from build123d import *

# Parameters (mm, degrees)
F1_DEPTH = 8
F2_W     = 118.303065
F2_H     = 130
F3_DEPTH = 2.5
F4_R     = 2.5
F5_DEPTH = 5


with BuildPart() as f1:
    # F0 (on Top) → F1 (new body)
    with BuildSketch(Plane.XY):
        with BuildLine():
            Line((-73, 0), (0, 0))
            Line((0, 0), (73, 0))
            ThreePointArc((73, 0), (74.414214, 0.585786), (75, 2))
            Line((75, 2), (75, 7.775523))
            ThreePointArc((75, 7.775523), (73.927452, 10.50133), (71.284988, 11.765358))
            Line((71.284988, 11.765358), (60.101284, 12.564194))
            ThreePointArc((60.101284, 12.564194), (55.064204, 13.247802), (50.154497, 14.564715))
            Line((50.154497, 14.564715), (16.502155, 25.927844))
            ThreePointArc((16.502155, 25.927844), (13.721064, 27.682003), (12.047716, 30.512454))
            ThreePointArc((12.047716, 30.512454), (11.731046, 31.611641), (11.450465, 32.720588))
            ThreePointArc((11.450465, 32.720588), (9.052802, 46.392588), (8.25, 60.25))
            Line((8.25, 60.25), (8.25, 92.25))
            ThreePointArc((8.25, 92.25), (9.052802, 106.107412), (11.450465, 119.779412))
            ThreePointArc((11.450465, 119.779412), (11.814902, 121.192928), (12.237963, 122.590018))
            ThreePointArc((12.237963, 122.590018), (13.860893, 125.287212), (16.501569, 127.000568))
            Line((16.501569, 127.000568), (35.134496, 133.776176))
            ThreePointArc((35.134496, 133.776176), (36.60869, 134.936374), (37.105525, 136.745369))
            Line((37.105525, 136.745369), (36.057795, 157.7))
            ThreePointArc((36.057795, 157.7), (35.86861, 159.074474), (35.444795, 160.395592))
            ThreePointArc((35.444795, 160.395592), (31.086723, 166.367805), (24.508944, 169.743151))
            ThreePointArc((24.508944, 169.743151), (18.300743, 170.974097), (12.006736, 171.63927))
            ThreePointArc((12.006736, 171.63927), (6.006077, 171.909797), (0, 172))
            ThreePointArc((0, 172), (-6.006077, 171.909797), (-12.006736, 171.63927))
            ThreePointArc((-12.006736, 171.63927), (-18.300743, 170.974097), (-24.508944, 169.743151))
            ThreePointArc((-24.508944, 169.743151), (-31.086723, 166.367805), (-35.444795, 160.395592))
            ThreePointArc((-35.444795, 160.395592), (-35.86861, 159.074474), (-36.057795, 157.7))
            Line((-36.057795, 157.7), (-37.105525, 136.745369))
            ThreePointArc((-37.105525, 136.745369), (-36.60869, 134.936374), (-35.134496, 133.776176))
            Line((-35.134496, 133.776176), (-16.501569, 127.000568))
            ThreePointArc((-16.501569, 127.000568), (-13.860893, 125.287212), (-12.237963, 122.590018))
            ThreePointArc((-12.237963, 122.590018), (-11.814902, 121.192928), (-11.450465, 119.779412))
            ThreePointArc((-11.450465, 119.779412), (-9.052802, 106.107412), (-8.25, 92.25))
            Line((-8.25, 92.25), (-8.25, 60.25))
            ThreePointArc((-8.25, 60.25), (-9.052802, 46.392588), (-11.450465, 32.720588))
            ThreePointArc((-11.450465, 32.720588), (-11.731046, 31.611641), (-12.047716, 30.512454))
            ThreePointArc((-12.047716, 30.512454), (-13.721064, 27.682003), (-16.502155, 25.927844))
            Line((-16.502155, 25.927844), (-50.154497, 14.564715))
            ThreePointArc((-50.154497, 14.564715), (-55.064204, 13.247802), (-60.101284, 12.564194))
            Line((-60.101284, 12.564194), (-71.284988, 11.765358))
            ThreePointArc((-71.284988, 11.765358), (-73.927452, 10.50133), (-75, 7.775523))
            Line((-75, 7.775523), (-75, 2))
            ThreePointArc((-75, 2), (-74.414214, 0.585786), (-73, 0))
        make_face()
    extrude(amount=F1_DEPTH)

    # F2 (on face) → F3 (cut)
    with BuildSketch(Plane.XY.offset(8)):
        with Locations((59.151532, 83)):
            Rectangle(F2_W, F2_H)
    extrude(amount=-F3_DEPTH, mode=Mode.SUBTRACT)

    # F4 (on face) → F5 (join)
    with BuildSketch(Plane.XY.offset(8)):
        with Locations((0, 10)):
            Circle(F4_R)
        with Locations((-13, 148)):
            Circle(F4_R)
    extrude(amount=F5_DEPTH)


solid = f1.part
CAD build for the part. Positions are in the model's coordinates, mm. A direction names the side the tool comes from. Give positions to 0.01 mm unless a question says otherwise; leave off trailing zeros. Write each loop counter-clockwise with the first axis right and the second up, starting at its lowest first coordinate (ties: lowest second). Pieces come first, ordered by that corner, then holes. Notation, with made-up numbers: (57, 66.5) - (105, 66.5) arc R6 cw to (105, 75.5) - close; hole circle Ø3 at (81, -35.5). An arc over 180 degrees is marked (long way). Put each result on its own line as item: value.
(1) Saw through at D-D (y = 22.5). List the corners of the cut face in (x, z).
Working result:
outline: (-26.65, 0) - (26.65, 0) - (26.65, 5.5) - (0, 5.5) - (0, 8) - (-26.65, 8) - close
(2) Saw through at C-C (y = 141.5). List the corners of the cut face in (x, z).
Working result:
outline: (-36.87, 0) - (36.87, 0) - (36.87, 5.5) - (0, 5.5) - (0, 8) - (-36.87, 8) - close
(3) Saw through at A-A (z = 10.75). List the corners of the cut face in (x, y).
Working result:
outline: circle Ø5 at (-13, 148); circle Ø5 at (0, 10)
(4) Pull direction Y, two halves, no side cores. Call faces 4 (the cylindrical face through (-0.54, 7.56, 10.46)), 5 (the flat face through (-65.61, 12.17, 3.94)), 6 (the flat face through (33.56, 20.17, 3.06)): released by +Y, released by -Y, zero draft, split by the parting line, or undercut.
Working result:
face 4: split by the parting line
face 5: released by +Y
face 6: undercut
(5) Saw through at B-B (x = -28). List the corners of the cut face in (y, z).
Working result:
outline: (0, 0) - (22.05, 0) - (22.05, 8) - (0, 8) - close; (131.18, 0) - (168.44, 0) - (168.44, 8) - (131.18, 8) - close
(6) Wall check: L1, parallel to Y at x = 12, z = 6.5; L2, parallel to Z at x = 6, y = 149; L3, parallel to Y at x = 16, z = 5. Give the ranges that are in metal, low to high.
Working result:
L1: 0 to 18, 148 to 171.64
L2: 0 to 8
L3: 0 to 26.12, 126.8 to 171.28
(7) Drop flat-ended pins along their axis: pin 1 Ø1.6 at (y, z) = (83.5, 3.5) entering from +X; pin 2 Ø2 at (x, z) = (12, 7) entering from +Y; pin 3 Ø1 at (y, z) = (91, 9) entering from +X; pin 4 Ø4 at (y, z) = (117.5, 4.5) entering from -X. Give the stop position or say it passes through.
Working result:
pin 1: x = 8.25
pin 2: y = 171.7
pin 3: through
pin 4: x = -11.38
(8) Tool access for faces 1 (the cylindrical face through (55.134, 13.234, 3.944)), 2 (the flat face through (8.25, 76, 3)), 3 (the flat face through (-33.093, 20.326, 3.944)): list every direction of +Z, -Z, +X, -X, +Y, -Y with a clear straight run to the whole face (end or side of a thin tool).
Working result:
face 1: +Z, -Z, +X, +Y
face 2: +Z, -Z, +X
face 3: +Z, -Z, -X
